Source: CAD feature listing. Evaluate the final solid. Frame: model axes, mm. Face numbers are marked on the shaded views. A direction names the side the tool comes from. Round coordinates to 2 decimals unless told otherwise and drop trailing zeros. Loops run counter-clockwise (first coordinate to the right, second up) from the corner with the lowest first, then second, coordinate; pieces in that order, holes last. Notation, with made-up numbers: (82, 58) -> (104, 58) arc R8 ccw to (104, 66) -> close; hole circle Ø2 at (60, -13). An arc over 180 degrees is marked (long way). Put each result on its own line as item: value. Start each with the question number.
1. Cut plane B-B (y = 41). Return the cut outline in (x, z).
2. Cut plane A-A (z = 20). State how many separate pieces and enclosed holes the cut face has, then the cut area to 3 significant figures.
3. Set-up query: the marked faces 1, 2, 3, 4 and 5. Return all of +Z, -Z, +X, -X, +Y, -Y with unobstructed straight access to the full face (end or side cutting, diameter ignored); none if empty.
4. Material intervals for L1, parallel to Y at x = 3, z = 14; L2, parallel to Y at x = 6, z = -6; L3, parallel to Y at x = 6, z = 12.5, sorted ascending.
5. Draft query along X for the marked faces 6, 7, 8 and 9. Return one class per face: pulls with the +X half, pulls with the -X half, needs draft (parallel to the pull), parting line crosses it, or undercut.
6. Contact query for flat-ended pins moving along their axis: pin 1 (1.5 mm diameter, centred on x = 8, y = 49, fed in from -Z); pin 2 (3.5 mm diameter, centred on x = 1, z = 16, fed in from +Y); pin 3 (3.5 mm diameter, centred on x = 13, z = 10.5, fed in from -Y). Output: stop coordinate, or through.
```python
from build123d import *

# Parameters (mm, degrees)
IZIM1_W                      = 50.7
IZIM1_H                      = 48.2
Y_KSEKLIK_EKSTR_ZYON1_DEPTH  = 26.7
IZIM2_R                      = 8.7
Y_KSEKLIK_EKSTR_ZYON2_DEPTH  = 0.5
Y_KSEKLIK_EKSTR_ZYON3_DEPTH  = 11.9
IZIM4_R                      = 16.5
Y_KSEKLIK_EKSTR_ZYON4_DEPTH  = 0.9
IZIM5_R                      = 18
Y_KSEKLIK_EKSTR_ZYON5_DEPTH  = 0.9
Y_KSEKLIK_EKSTR_ZYON6_DEPTH  = 36
Y_KSEKLIK_EKSTR_ZYON7_DEPTH  = 17
Y_KSEKLIK_EKSTR_ZYON8_START  = 17
Y_KSEKLIK_EKSTR_ZYON8_DEPTH  = 17
IZIM9_W                      = 14.75
IZIM9_H                      = 70
KES_EKSTR_ZYON1_DEPTH        = 30.160746911
IZIM10_W                     = 14.75
IZIM10_H                     = 70
KES_EKSTR_ZYON2_DEPTH        = 30.160746911
IZIM11_W                     = 50.7
IZIM11_H                     = 48.2
Y_KSEKLIK_EKSTR_ZYON9_DEPTH  = 9.3
Y_KSEKLIK_EKSTR_ZYON10_START = 20
Y_KSEKLIK_EKSTR_ZYON10_DEPTH = 20
IZIM13_W                     = 9.75
IZIM13_H                     = 10.2
Y_KSEKLIK_EKSTR_ZYON11_DEPTH = 26.5
Y_KSEKLIK_EKSTR_ZYON12_DEPTH = 42.2
Y_KSEKLIK_EKSTR_ZYON13_START = -42.2
Y_KSEKLIK_EKSTR_ZYON13_DEPTH = 42.2
IZIM16_W                     = 29
IZIM16_H                     = 34.79
Y_KSEKLIK_EKSTR_ZYON14_DEPTH = 9.9
Y_KSEKLIK_EKSTR_ZYON15_DEPTH = 8.5
Y_KSEKLIK_EKSTR_ZYON16_DEPTH = 8.5
IZIM19_W                     = 6.3
IZIM19_H                     = 0.8
Y_KSEKLIK_EKSTR_ZYON17_DEPTH = 12
DRAFT1_ANGLE                 = 50
IZIM20_W                     = 5
IZIM20_H                     = 7.5
IZIM21_W                     = 5
IZIM21_H                     = 7.5
IZIM22_W                     = 5
IZIM22_H                     = 7.5
IZIM23_W                     = 5
IZIM23_H                     = 7.5
IZIM24_W                     = 5.2
IZIM24_H                     = 2.6
M27_BO_LUKLU_DELIK1_D        = 30.291
M27_BO_LUKLU_DELIK1_DEPTH    = 33.249
M27_BO_LUKLU_DELIK2_D        = 30.291
M27_BO_LUKLU_DELIK2_DEPTH    = 33.249
FEDER1_START                 = -30
FEDER1_DEPTH                 = 9.75
PAH1_SIZE                    = 1.479
RADYUS1_R                    = 0.8
RADYUS2_R                    = 2
RADYUS3_R                    = 5
RADYUS4_R                    = 5.1
RADYUS5_R                    = 7
RADYUS6_R                    = 8.16
L_EK1_SCALE                  = 0.46


# Read off the part's stored shape, not the designer's step: Feder1
with BuildPart() as part:
    # Çizim1 → Yükseklik-Ekstrüzyon1 (new body)
    with BuildSketch(Plane(origin=(18, 0, 0), x_dir=(0, 0, -1), z_dir=(1, 0, 0))):
        with Locations((-0.35, 68.8)):
            Rectangle(IZIM1_W, IZIM1_H)
    extrude(amount=-Y_KSEKLIK_EKSTR_ZYON1_DEPTH)

    # Çizim2 → Yükseklik-Ekstrüzyon2 (add)
    with BuildSketch(Plane.XZ.offset(-44.7)):
        with Locations(Location((0, 0, 0), (0, 0, 180))):
            Circle(IZIM2_R)
    extrude(amount=Y_KSEKLIK_EKSTR_ZYON2_DEPTH)

    # Çizim3 → Yükseklik-Ekstrüzyon3 (add)
    with BuildSketch(Plane(origin=(0, 44.2, 0), x_dir=(1, 0, 0), z_dir=(0, 1, 0))):
        Polygon((-18, 10.392304845), (-18, -10.392304845), (0, -20.784609691), (18, -10.392304845), (18, 10.392304845), (0, 20.784609691), align=None)
    extrude(amount=-Y_KSEKLIK_EKSTR_ZYON3_DEPTH)

    # Çizim4 → Yükseklik-Ekstrüzyon4 (add)
    with BuildSketch(Plane.XZ.offset(-32.3)):
        with Locations(Location((0, 0, 0), (0, 0, 270))):
            Circle(IZIM4_R)
    extrude(amount=Y_KSEKLIK_EKSTR_ZYON4_DEPTH)

    # Çizim5 → Yükseklik-Ekstrüzyon5 (add)
    with BuildSketch(Plane(origin=(0, 31.4, 0), x_dir=(1, 0, 0), z_dir=(0, 1, 0))):
        with Locations(Location((0, 0, 0), (0, 0, 90))):
            Circle(IZIM5_R)
    extrude(amount=-Y_KSEKLIK_EKSTR_ZYON5_DEPTH)

    # Çizim6 → Yükseklik-Ekstrüzyon6 (add)
    with BuildSketch(Plane.XY.offset(18)):
        with BuildLine():
            Line((-13.564659966, -21), (13.564659966, -21))
            ThreePointArc((13.564659966, -21), (17.201870235, -18.14099392), (20.25, -14.660746911))
            Line((20.25, -14.660746911), (35, -14.660746911))
            Line((35, -14.660746911), (35, 30.5))
            Line((35, 30.5), (0, 30.5))
            Line((0, 30.5), (-35, 30.5))
            Line((-35, 30.5), (-35, -14.660746911))
            Line((-35, -14.660746911), (-20.25, -14.660746911))
            ThreePointArc((-20.25, -14.660746911), (-17.201870235, -18.14099392), (-13.564659966, -21))
        make_face()
    extrude(amount=-Y_KSEKLIK_EKSTR_ZYON6_DEPTH)

    # Çizim7 → Yükseklik-Ekstrüzyon7 (add)
    with BuildSketch(Plane(origin=(0, 0, -18), x_dir=(-1, 0, 0), z_dir=(0, 0, -1))):
        with BuildLine():
            Line((13.564659966, -21), (-13.564659966, -21))
            ThreePointArc((-13.564659966, -21), (-17.201870235, -18.14099392), (-20.25, -14.660746911))
            Line((-20.25, -14.660746911), (-35, -14.660746911))
            Line((-35, -14.660746911), (-35, 30.5))
            Line((-35, 30.5), (35, 30.5))
            Line((35, 30.5), (35, -14.660746911))
            Line((35, -14.660746911), (20.25, -14.660746911))
            ThreePointArc((20.25, -14.660746911), (17.201870235, -18.14099392), (13.564659966, -21))
        make_face()
    extrude(amount=Y_KSEKLIK_EKSTR_ZYON7_DEPTH)

    # Çizim8 → Yükseklik-Ekstrüzyon8 (add)
    with BuildSketch(Plane.XY.offset(18).offset(Y_KSEKLIK_EKSTR_ZYON8_START)):
        with BuildLine():
            Line((13.564659966, -21), (-13.564659966, -21))
            ThreePointArc((-13.564659966, -21), (-17.201870235, -18.14099392), (-20.25, -14.660746911))
            Line((-20.25, -14.660746911), (-35, -14.660746911))
            Line((-35, -14.660746911), (-35, 30.5))
            Line((-35, 30.5), (35, 30.5))
            Line((35, 30.5), (35, -14.660746911))
            Line((35, -14.660746911), (20.25, -14.660746911))
            ThreePointArc((20.25, -14.660746911), (17.201870235, -18.14099392), (13.564659966, -21))
        make_face()
    extrude(amount=-Y_KSEKLIK_EKSTR_ZYON8_DEPTH)

    # Çizim9 → Kes-Ekstrüzyon1 (cut)
    with BuildSketch(Plane.XZ.offset(14.660746911)):
        with Locations((27.625, 0)):
            Rectangle(IZIM9_W, IZIM9_H)
    extrude(amount=-KES_EKSTR_ZYON1_DEPTH, mode=Mode.SUBTRACT)

    # Çizim10 → Kes-Ekstrüzyon2 (cut)
    with BuildSketch(Plane.XZ.offset(14.660746911)):
        with Locations((-27.625, 0)):
            Rectangle(IZIM10_W, IZIM10_H)
    extrude(amount=-KES_EKSTR_ZYON2_DEPTH, mode=Mode.SUBTRACT)

    # Çizim11 → Yükseklik-Ekstrüzyon9 (add)
    with BuildSketch(Plane.ZY.offset(8.7)):
        with Locations((0.35, 68.8)):
            Rectangle(IZIM11_W, IZIM11_H)
    extrude(amount=Y_KSEKLIK_EKSTR_ZYON9_DEPTH)

    # Çizim12 → Yükseklik-Ekstrüzyon10 (add)
    with BuildSketch(Plane.XY.offset(35).offset(Y_KSEKLIK_EKSTR_ZYON10_START)):
        with BuildLine():
            Line((-20.25, -14.660746911), (-20.25, 17.715834237))
            ThreePointArc((-20.25, 17.715834237), (0, 22), (20.25, 17.715834237))
            Line((20.25, 17.715834237), (20.25, -14.660746911))
            ThreePointArc((20.25, -14.660746911), (17.201870235, -18.14099392), (13.564659966, -21))
            Line((13.564659966, -21), (-13.564659966, -21))
            ThreePointArc((-13.564659966, -21), (-17.201870235, -18.14099392), (-20.25, -14.660746911))
        make_face()
    extrude(amount=-Y_KSEKLIK_EKSTR_ZYON10_DEPTH)

    # Çizim13 → Yükseklik-Ekstrüzyon11 (add)
    with BuildSketch(Plane.XZ.offset(-15.5)):
        with Locations((25.125, 15.1)):
            Rectangle(IZIM13_W, IZIM13_H)
    extrude(amount=Y_KSEKLIK_EKSTR_ZYON11_DEPTH)

    # Çizim14 → Yükseklik-Ekstrüzyon12 (add)
    with BuildSketch(Plane(origin=(0, 89.9, 0), x_dir=(1, 0, 0), z_dir=(0, 1, 0))):
        with BuildLine():
            Line((-18, -8.717797887), (-18, 8.717797887))
            ThreePointArc((-18, 8.717797887), (-20, 0), (-18, -8.717797887))
        make_face()
    extrude(amount=-Y_KSEKLIK_EKSTR_ZYON12_DEPTH)

    # Çizim15 → Yükseklik-Ekstrüzyon13 (add)
    with BuildSketch(Plane.XZ.offset(-47.7).offset(Y_KSEKLIK_EKSTR_ZYON13_START)):
        with BuildLine():
            Line((18, 8.717797887), (18, -8.717797887))
            ThreePointArc((18, -8.717797887), (20, 0), (18, 8.717797887))
        make_face()
    extrude(amount=Y_KSEKLIK_EKSTR_ZYON13_DEPTH)

    # Çizim16 → Yükseklik-Ekstrüzyon14 (add)
    with BuildSketch(Plane.XY.offset(25.7)):
        with Locations((0, 75.495)):
            Rectangle(IZIM16_W, IZIM16_H)
    extrude(amount=Y_KSEKLIK_EKSTR_ZYON14_DEPTH)

    # Çizim17 → Yükseklik-Ekstrüzyon15 (add)
    with BuildSketch(Plane.XY.offset(35.6)):
        Polygon((-9.4, 81.4), (-7.6, 81.4), (-7.6, 80.6), (-8.6, 80.6), (-8.6, 77.4), (-7.6, 77.4), (-7.6, 76.6), (-9.4, 76.6), align=None)
    extrude(amount=Y_KSEKLIK_EKSTR_ZYON15_DEPTH)

    # Çizim18 → Yükseklik-Ekstrüzyon16 (add)
    with BuildSketch(Plane.XY.offset(35.6)):
        Polygon((7.6, 77.4), (8.6, 77.4), (8.6, 80.6), (7.6, 80.6), (7.6, 81.4), (9.4, 81.4), (9.4, 76.6), (7.6, 76.6), align=None)
    extrude(amount=Y_KSEKLIK_EKSTR_ZYON16_DEPTH)

    # Çizim19 → Yükseklik-Ekstrüzyon17 (add)
    with BuildSketch(Plane.XY.offset(35.6)):
        with Locations((0, 70)):
            Rectangle(IZIM19_W, IZIM19_H)
    extrude(amount=Y_KSEKLIK_EKSTR_ZYON17_DEPTH)

    # Draft1
    draft1_faces = [part.faces().sort_by_distance(p)[0] for p in [
        (25.125, 2.25, 10),
    ]]
    draft(draft1_faces, Plane(origin=(0, -11, 0), x_dir=(0, 0, -1), z_dir=(0, -1, 0)), DRAFT1_ANGLE)

    # Çizim20 → Döndür1 (revolve)
    with BuildSketch(Plane.XY.offset(26.25), mode=Mode.PRIVATE) as d_nd_r1_sk:
        with Locations((-23.75, 34.25)):
            Rectangle(IZIM20_W, IZIM20_H)
    revolve(d_nd_r1_sk.sketch.rotate(Axis((-26.25, 38, 26.25), (0, -1, 0)), 270), axis=Axis((-26.25, 38, 26.25), (0, -1, 0)))

    # Çizim21 → Döndür2 (revolve)
    with BuildSketch(Plane.XY.offset(-26.25), mode=Mode.PRIVATE) as d_nd_r2_sk:
        with Locations((-23.75, 34.25)):
            Rectangle(IZIM21_W, IZIM21_H)
    revolve(d_nd_r2_sk.sketch.rotate(Axis((-26.25, 38, -26.25), (0, -1, 0)), 270), axis=Axis((-26.25, 38, -26.25), (0, -1, 0)))

    # Çizim22 → Döndür3 (revolve)
    with BuildSketch(Plane.XY.offset(-26.25), mode=Mode.PRIVATE) as d_nd_r3_sk:
        with Locations((28.75, 34.25)):
            Rectangle(IZIM22_W, IZIM22_H)
    revolve(d_nd_r3_sk.sketch.rotate(Axis((26.25, 38, -26.25), (0, -1, 0)), 270), axis=Axis((26.25, 38, -26.25), (0, -1, 0)))

    # Çizim23 → Döndür4 (revolve)
    with BuildSketch(Plane.XY.offset(26.25), mode=Mode.PRIVATE) as d_nd_r4_sk:
        with Locations((28.75, 34.25)):
            Rectangle(IZIM23_W, IZIM23_H)
    revolve(d_nd_r4_sk.sketch.rotate(Axis((26.25, 38, 26.25), (0, -1, 0)), 270), axis=Axis((26.25, 38, 26.25), (0, -1, 0)))

    # Çizim24 → Döndür5 (revolve)
    with BuildSketch(Plane(origin=(0, 0, 0), x_dir=(-1, 0, 0), z_dir=(0, 0, -1)), mode=Mode.PRIVATE) as d_nd_r5_sk:
        with Locations((-2.6, 94.2)):
            Rectangle(IZIM24_W, IZIM24_H)
    revolve(d_nd_r5_sk.sketch.rotate(Axis((0, 92.9, 0), (0, 1, 0)), 90), axis=Axis((0, 92.9, 0), (0, 1, 0)))

    # M27 Boşluklu Delik1
    with Locations(Plane.XY.offset(55)):
        with Locations((0, 0)):
            Hole(M27_BO_LUKLU_DELIK1_D / 2, depth=M27_BO_LUKLU_DELIK1_DEPTH)

    # M27 Boşluklu Delik2
    with Locations(Plane(origin=(0, 0, -35), x_dir=(-1, 0, 0), z_dir=(0, 0, -1))):
        with Locations((0, 0)):
            Hole(M27_BO_LUKLU_DELIK2_D / 2, depth=M27_BO_LUKLU_DELIK2_DEPTH)

    # Feder1 outline → Feder1 (add)
    with BuildSketch(Plane.YZ.offset(FEDER1_START)):
        Polygon((15.5, 19.826070485), (-9.313312955, 19.826070485), (-12.686687045, 12.591846402), (15.5, -20.999739147), align=None)
    extrude(amount=FEDER1_DEPTH)

    # Pah1
    pah1_edges = [part.edges().sort_by_distance(p)[0] for p in [
        (15.1455, 0, 55),
        (-15.1455, 0, -35),
    ]]
    chamfer(pah1_edges, length=PAH1_SIZE)

    # Radyus1
    radyus1_edges = [part.edges().sort_by_distance(p)[0] for p in [
        (-9.4, 81.4, 39.85),
        (-9.4, 76.6, 39.85),
        (9.4, 76.6, 39.85),
        (9.4, 81.4, 39.85),
    ]]
    fillet(radyus1_edges, radius=RADYUS1_R)

    # Radyus2
    radyus2_edges = [part.edges().sort_by_distance(p)[0] for p in [
        (-18, 68.8, -25),
        (-18, 68.8, 25.7),
        (-14.5, 92.89, 30.65),
        (-14.5, 58.1, 30.65),
        (14.5, 58.1, 30.65),
        (14.5, 92.89, 30.65),
        (18, 68.8, 25.7),
        (18, 68.8, -25),
    ]]
    fillet(radyus2_edges, radius=RADYUS2_R)

    # Radyus3
    radyus3_edges = [part.edges().sort_by_distance(p)[0] for p in [
        (-18, 38.25, -10.392304845),
        (0, 38.25, -20.784609691),
        (18, 38.25, -10.392304845),
        (18, 38.25, 10.392304845),
        (0, 38.25, 20.784609691),
        (-18, 38.25, 10.392304845),
    ]]
    fillet(radyus3_edges, radius=RADYUS3_R)

    # Radyus4
    radyus4_edges = [part.edges().sort_by_distance(p)[0] for p in [
        (25.125, -11, 20.2),
    ]]
    fillet(radyus4_edges, radius=RADYUS4_R)

    # Radyus5
    radyus5_edges = [part.edges().sort_by_distance(p)[0] for p in [
        (35, 23, 35),
        (-35, 23, -35),
        (35, 23, -35),
        (-35, 23, 35),
    ]]
    fillet(radyus5_edges, radius=RADYUS5_R)

    # Radyus6
    radyus6_edges = [part.edges().sort_by_distance(p)[0] for p in [
        (25.125, -11, 10),
    ]]
    fillet(radyus6_edges, radius=RADYUS6_R)


with BuildPart() as part_1:
    # Ölçek1: scaled about (0.014445195, 31.538640435, 4.897050437)
    add(part.part.scale(L_EK1_SCALE).moved(Location((0.007800405, 17.030865835, 2.644407236))))


solid = part_1.part
```
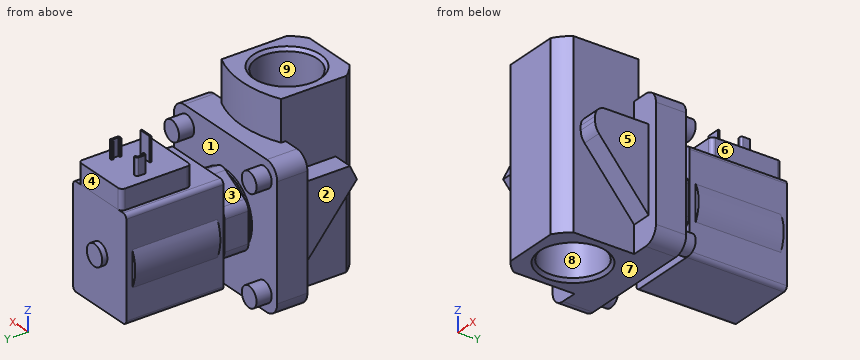
Solution:
1. outline: (-8.27, -7.94) arc R0.92 ccw to (-7.35, -8.86) -> (7.37, -8.86) arc R0.92 ccw to (8.29, -7.94) -> (8.29, -1.37) arc R9.2 ccw to (8.29, 6.65) -> (8.29, 13.55) arc R0.92 ccw to (7.37, 14.47) -> (-7.35, 14.47) arc R0.92 ccw to (-8.27, 13.55) -> (-8.27, 6.65) arc R9.2 ccw to (-8.27, -1.37) -> close
2. separate pieces: 4
2. enclosed holes: 1
2. area: 199 mm^2
3. face 1: none
3. face 2: +Z, -Z, -X, -Y
3. face 3: +Z, -X
3. face 4: +Z, +X, -X, +Y
3. face 5: +Z, -Z, +X, -Y
4. L1: y = 7.37 to 10.74, 23.32 to 31.06, 37.59 to 59.76
4. L2: y = 7.37 to 13.48, 20.58 to 31.06, 37.59 to 59.76
4. L3: y = 7.37 to 31.06, 37.59 to 59.76
5. face 6: pulls with the +X half
5. face 7: needs draft
5. face 8: undercut
5. face 9: undercut
6. pin 1: stops at z = -8.86
6. pin 2: stops at y = 59.76
6. pin 3: stops at y = 11.97
